Design review of the part built by this model. Coordinates are the model's own, in mm. A direction names the side the tool comes from. Coordinates: 2 decimals unless noted, no trailing zeros. Loops run counter-clockwise (first coordinate to the right, second up) from the corner with the lowest first, then second, coordinate; pieces in that order, holes last. Notation, with made-up numbers: M 16,23 L 55,23 A19 ccw 55,43 Z; hole C 19,32.25 d3. An arc over 180 degrees is marked long. Put each result on its own line as item: value. Start each with the question number.
(1) The part is to be moulded in two halves that separate along X. For faces 5 (the flat face through (5.9, 22, 11)), 6 (the flat face through (9, 17.5, 11)), 7 (the flat face through (-10, 0, 10)), say which applies: +X half, -X half, draft (parallel to the pull), parting line (faces both ways), or undercut.
(2) Take a section at D-D, the plane y = -14. Give the boundary of the cut face in (x, z).
(3) Clearance check with flat-ended pins moving along their axes: pin 1 (1 mm diameter, centred on x = -8.5, z = 11.5, fed in from +Y); pin 2 (0.6 mm diameter, centred on x = -9.5, z = 12.5, fed in from +Y); pin 3 (0.6 mm diameter, centred on x = -8.5, z = 9, fed in from -Y). State where each tip first meets the part, or that it passes through.
(4) For faces 1 (the flat face through (9, 18, 3)), 2 (the flat face through (-7.5, 17, 19)), 3 (the flat face through (-9, 14, 3)), 4 (the cylindrical face through (2.064, 12.392, 9.915)), list the 3-axis set-ups (+Z, -Z, +X, -X, +Y, -Y) from which the entire face can be reached by the end or side of a thin tool; tool diameter is ignored.
(5) For probe 1 along Y at (x, z) = (0, 8.5); probe 2 along Y at (x, z) = (-1.5, 6); probe 3 along X at (y, z) = (-8, 10), list the stretches that pass through material, from the lowest coordinate up. Write a range as [from, to].
(6) Take a section at A-A, the plane y = 10.5. Give the boundary of the cut face in (x, z).
(7) Take a section at C-C, the plane z = 12.75. Count the separate pieces of the cut face and the enclosed holes in it, then the cut area to 3 significant figures.
(8) Take a section at B-B, the plane x = 0. Give the boundary of the cut face in (y, z), then the cut area to 3 significant figures.
```python
from build123d import *

# Parameters (mm, degrees)
SKETCH2_W           = 20
SKETCH2_H           = 45
BOSS_EXTRUDE1_DEPTH = 20
SHELL1_T            = -2
CUT_EXTRUDE1_REACH  = 38.142
SKETCH3_W           = 15
SKETCH3_H           = 2
CUT_EXTRUDE2_REACH  = 52.249
SKETCH4_W           = 2
SKETCH4_H           = 15
FILLET1_R           = 3
SKETCH7_W           = 15
SKETCH7_H           = 3
CUT_EXTRUDE3_DEPTH  = 2
FILLET3_R           = 0.5
SKETCH8_R           = 5.2
SKETCH8_R_2         = 2.8
BOSS_EXTRUDE2_DEPTH = 16.4


with BuildPart() as part:
    # Sketch2 → Boss-Extrude1 (new body)
    with BuildSketch(Plane.XY):
        Rectangle(SKETCH2_W, SKETCH2_H)
    extrude(amount=BOSS_EXTRUDE1_DEPTH)

    # Shell1
    shell1_openings = [part.faces().sort_by_distance(p)[0] for p in [
        (0, 0, 0),
    ]]
    offset(amount=SHELL1_T, openings=shell1_openings, kind=Kind.INTERSECTION)

    # Cut-Extrude1: up to this face of the body (flat: up to its plane)
    cut_extrude1_end = Plane(part.part.faces().sort_by_distance((-10, 0, 10))[0])
    # Sketch3 → Cut-Extrude1 (cut, up to the picked face)
    with BuildSketch(Plane(origin=(10, 0, 0), x_dir=(0, 0, -1), z_dir=(1, 0, 0)), mode=Mode.PRIVATE) as cut_extrude1_sk1:
        with Locations((-10.5, 18.5)):
            Rectangle(SKETCH3_W, SKETCH3_H)
    cut_extrude1_tool1 = split(extrude(cut_extrude1_sk1.sketch, amount=-CUT_EXTRUDE1_REACH, mode=Mode.PRIVATE), bisect_by=cut_extrude1_end, keep=Keep.BOTH, mode=Mode.PRIVATE)
    # Sketch3 → Cut-Extrude1 (cut, up to the picked face)
    with BuildSketch(Plane(origin=(10, 0, 0), x_dir=(0, 0, -1), z_dir=(1, 0, 0)), mode=Mode.PRIVATE) as cut_extrude1_sk2:
        with Locations((-10.5, 14.5)):
            Rectangle(SKETCH3_W, SKETCH3_H)
    cut_extrude1_tool2 = split(extrude(cut_extrude1_sk2.sketch, amount=-CUT_EXTRUDE1_REACH, mode=Mode.PRIVATE), bisect_by=cut_extrude1_end, keep=Keep.BOTH, mode=Mode.PRIVATE)
    # Sketch3 → Cut-Extrude1 (cut, up to the picked face)
    with BuildSketch(Plane(origin=(10, 0, 0), x_dir=(0, 0, -1), z_dir=(1, 0, 0)), mode=Mode.PRIVATE) as cut_extrude1_sk3:
        with Locations((-10.5, 10.5)):
            Rectangle(SKETCH3_W, SKETCH3_H)
    cut_extrude1_tool3 = split(extrude(cut_extrude1_sk3.sketch, amount=-CUT_EXTRUDE1_REACH, mode=Mode.PRIVATE), bisect_by=cut_extrude1_end, keep=Keep.BOTH, mode=Mode.PRIVATE)
    # Sketch3 → Cut-Extrude1 (cut, up to the picked face)
    with BuildSketch(Plane(origin=(10, 0, 0), x_dir=(0, 0, -1), z_dir=(1, 0, 0)), mode=Mode.PRIVATE) as cut_extrude1_sk4:
        with Locations((-10.5, 6.5)):
            Rectangle(SKETCH3_W, SKETCH3_H)
    cut_extrude1_tool4 = split(extrude(cut_extrude1_sk4.sketch, amount=-CUT_EXTRUDE1_REACH, mode=Mode.PRIVATE), bisect_by=cut_extrude1_end, keep=Keep.BOTH, mode=Mode.PRIVATE)
    # Sketch3 → Cut-Extrude1 (cut, up to the picked face)
    with BuildSketch(Plane(origin=(10, 0, 0), x_dir=(0, 0, -1), z_dir=(1, 0, 0)), mode=Mode.PRIVATE) as cut_extrude1_sk5:
        with Locations((-10.5, 2.5)):
            Rectangle(SKETCH3_W, SKETCH3_H)
    cut_extrude1_tool5 = split(extrude(cut_extrude1_sk5.sketch, amount=-CUT_EXTRUDE1_REACH, mode=Mode.PRIVATE), bisect_by=cut_extrude1_end, keep=Keep.BOTH, mode=Mode.PRIVATE)
    # Sketch3 → Cut-Extrude1 (cut, up to the picked face)
    with BuildSketch(Plane(origin=(10, 0, 0), x_dir=(0, 0, -1), z_dir=(1, 0, 0)), mode=Mode.PRIVATE) as cut_extrude1_sk6:
        with Locations((-10.5, -1.5)):
            Rectangle(SKETCH3_W, SKETCH3_H)
    cut_extrude1_tool6 = split(extrude(cut_extrude1_sk6.sketch, amount=-CUT_EXTRUDE1_REACH, mode=Mode.PRIVATE), bisect_by=cut_extrude1_end, keep=Keep.BOTH, mode=Mode.PRIVATE)
    add(cut_extrude1_tool1.solids().sort_by(Axis((10, 18.5, 10.5), (-1, 0, 0)))[0], mode=Mode.SUBTRACT)
    add(cut_extrude1_tool2.solids().sort_by(Axis((10, 14.5, 10.5), (-1, 0, 0)))[0], mode=Mode.SUBTRACT)
    add(cut_extrude1_tool3.solids().sort_by(Axis((10, 10.5, 10.5), (-1, 0, 0)))[0], mode=Mode.SUBTRACT)
    add(cut_extrude1_tool4.solids().sort_by(Axis((10, 6.5, 10.5), (-1, 0, 0)))[0], mode=Mode.SUBTRACT)
    add(cut_extrude1_tool5.solids().sort_by(Axis((10, 2.5, 10.5), (-1, 0, 0)))[0], mode=Mode.SUBTRACT)
    add(cut_extrude1_tool6.solids().sort_by(Axis((10, -1.5, 10.5), (-1, 0, 0)))[0], mode=Mode.SUBTRACT)

    # Sketch4 → Cut-Extrude2 (cut, up to next)
    with BuildSketch(Plane(origin=(0, 22.5, 0), x_dir=(1, 0, 0), z_dir=(0, 1, 0)), mode=Mode.PRIVATE) as cut_extrude2_sk1:
        with Locations((-6.9, -10.5)):
            Rectangle(SKETCH4_W, SKETCH4_H)
    cut_extrude2_tool1 = extrude(cut_extrude2_sk1.sketch, amount=-CUT_EXTRUDE2_REACH, mode=Mode.PRIVATE) & part.part
    # Sketch4 → Cut-Extrude2 (cut, up to next)
    with BuildSketch(Plane(origin=(0, 22.5, 0), x_dir=(1, 0, 0), z_dir=(0, 1, 0)), mode=Mode.PRIVATE) as cut_extrude2_sk2:
        with Locations((-2.3, -10.5)):
            Rectangle(SKETCH4_W, SKETCH4_H)
    cut_extrude2_tool2 = extrude(cut_extrude2_sk2.sketch, amount=-CUT_EXTRUDE2_REACH, mode=Mode.PRIVATE) & part.part
    # Sketch4 → Cut-Extrude2 (cut, up to next)
    with BuildSketch(Plane(origin=(0, 22.5, 0), x_dir=(1, 0, 0), z_dir=(0, 1, 0)), mode=Mode.PRIVATE) as cut_extrude2_sk3:
        with Locations((2.3, -10.5)):
            Rectangle(SKETCH4_W, SKETCH4_H)
    cut_extrude2_tool3 = extrude(cut_extrude2_sk3.sketch, amount=-CUT_EXTRUDE2_REACH, mode=Mode.PRIVATE) & part.part
    # Sketch4 → Cut-Extrude2 (cut, up to next)
    with BuildSketch(Plane(origin=(0, 22.5, 0), x_dir=(1, 0, 0), z_dir=(0, 1, 0)), mode=Mode.PRIVATE) as cut_extrude2_sk4:
        with Locations((6.9, -10.5)):
            Rectangle(SKETCH4_W, SKETCH4_H)
    cut_extrude2_tool4 = extrude(cut_extrude2_sk4.sketch, amount=-CUT_EXTRUDE2_REACH, mode=Mode.PRIVATE) & part.part
    add(cut_extrude2_tool1.solids().sort_by_distance((-6.9, 22.5, 10.5))[0], mode=Mode.SUBTRACT)
    add(cut_extrude2_tool2.solids().sort_by_distance((-2.3, 22.5, 10.5))[0], mode=Mode.SUBTRACT)
    add(cut_extrude2_tool3.solids().sort_by_distance((2.3, 22.5, 10.5))[0], mode=Mode.SUBTRACT)
    add(cut_extrude2_tool4.solids().sort_by_distance((6.9, 22.5, 10.5))[0], mode=Mode.SUBTRACT)

    # Fillet1
    # the kernel refuses this fillet: 3 mm, written as the material it takes off along each edge
    with BuildSketch(Plane(origin=(10, -22.5, -7.5), x_dir=(-1, 0, 0), z_dir=(0, 0, 1)), Plane(origin=(10, 22.5, -7.5), x_dir=(0, -1, 0), z_dir=(0, 0, 1))) as fillet1_piece_1:
        with BuildLine():
            CenterArc((FILLET1_R, -FILLET1_R), FILLET1_R, 90, 90)
            Line((0, -FILLET1_R), (0, 0))
            Line((0, 0), (FILLET1_R, 0))
        make_face()
    extrude(amount=35, mode=Mode.SUBTRACT)
    with BuildSketch(Plane(origin=(-10, -22.5, -7.5), x_dir=(1, 0, 0), z_dir=(0, 0, 1)), Plane(origin=(-10, 22.5, -7.5), x_dir=(0, -1, 0), z_dir=(0, 0, 1))) as fillet1_piece_2:
        with BuildLine():
            CenterArc((FILLET1_R, FILLET1_R), FILLET1_R, 180, 90)
            Line((0, FILLET1_R), (0, 0))
            Line((0, 0), (FILLET1_R, 0))
        make_face()
    extrude(amount=35, mode=Mode.SUBTRACT)

    # Sketch7 → Cut-Extrude3 (cut)
    with BuildSketch(Plane.XY.offset(20)):
        with Locations((0, 17.5)):
            Rectangle(SKETCH7_W, SKETCH7_H)
    extrude(amount=-CUT_EXTRUDE3_DEPTH, mode=Mode.SUBTRACT)

    # Fillet3
    fillet3_edges = [part.edges().sort_by_distance(p)[0] for p in [
        (10, 0, 20),
        (0, -22.5, 20),
        (-10, 0, 20),
        (0, 22.5, 20),
        (9.121320344, 21.621320344, 20),
        (-9.121320344, 21.621320344, 20),
        (-9.121320344, -21.621320344, 20),
        (9.121320344, -21.621320344, 20),
    ]]
    fillet(fillet3_edges, radius=FILLET3_R)

    # Sketch8 → Boss-Extrude2 (add)
    with BuildSketch(Plane(origin=(0, 0, 18), x_dir=(-1, 0, 0), z_dir=(0, 0, -1))):
        with Locations(Location((0, 10.5, 0), (0, 0, 180))):
            Circle(SKETCH8_R)
        with Locations((0, 10.5)):
            Circle(SKETCH8_R_2, mode=Mode.SUBTRACT)
    extrude(amount=BOSS_EXTRUDE2_DEPTH)


solid = part.part
```
Computed values:
1. face 5: undercut
1. face 6: draft
1. face 7: -X half
2. outline: M -10,0 L -8,0 L -8,18 L 8,18 L 8,0 L 10,0 L 10,19.5 A0.5 ccw 9.5,20 L -9.5,20 A0.5 ccw -10,19.5 Z
3. pin 1: stops at y = 22.33
3. pin 2: stops at y = 21.54
3. pin 3: stops at y = -22.25
4. face 1: +X, -X
4. face 2: +Z, -Z
4. face 3: -X
4. face 4: -Z
5. probe 1: y = [-22.5, -20.5], [5.3, 7.7], [13.3, 15.7], [20.5, 22.5]
5. probe 2: y = [-22.5, -20.5], [5.52, 8.14], [12.86, 15.48]
5. probe 3: x = [-10, -8], [8, 10]
6. outline: M -10,0 L -8,0 L -8,3 L -10,3 Z; M -10,18 L -5.2,18 L -5.2,1.6 L -2.8,1.6 L -2.8,18 L 2.8,18 L 2.8,1.6 L 5.2,1.6 L 5.2,18 L 10,18 L 10,19.5 A0.5 ccw 9.5,20 L -9.5,20 A0.5 ccw -10,19.5 Z; M 8,0 L 10,0 L 10,3 L 8,3 Z
7. separate pieces: 17
7. enclosed holes: 1
7. area: 233 mm^2
8. outline: M -22.5,0 L -20.5,0 L -20.5,18 L 5.3,18 L 5.3,1.6 L 7.7,1.6 L 7.7,18 L 13.3,18 L 13.3,1.6 L 15.7,1.6 L 15.7,18 L 16,18 L 16,20 L -22,20 A0.5 ccw -22.5,19.5 Z; M 19,18 L 20.5,18 L 20.5,0 L 22.5,0 L 22.5,19.5 A0.5 ccw 22,20 L 19,20 Z
8. area: 235 mm^2
